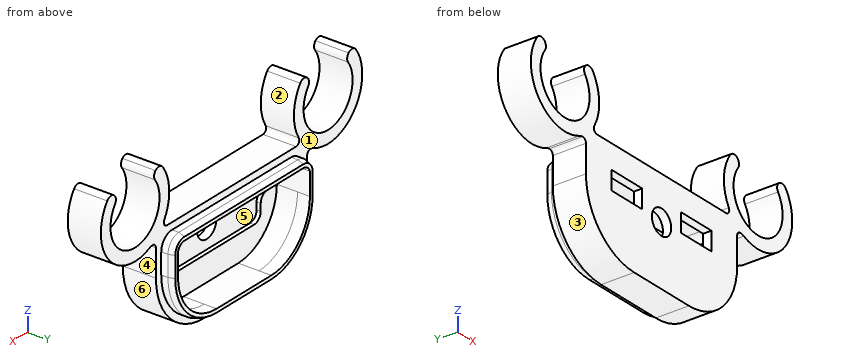
```python
from build123d import *

# Parameters (mm, degrees)
SKETCH1_W               = 47
SKETCH1_H               = 25
BOSS_EXTRUDE1_DEPTH     = 8
SHELL1_T                = -3
SKETCH4_R               = 3
SKETCH4_W               = 9.5
SKETCH4_H               = 4.5
CUT_EXTRUDE4_DEPTH      = 28.793884219
FILLET2_R               = 12
FILLET3_R               = 15
SKETCH5_R               = 7.625
BOSS_EXTRUDE3_DEPTH     = 8
FILLET7_R               = 2
FILLET9_R               = 3
FILLET10_R              = 3
BOSS_EXTRUDE4_DEPTH     = 3
FILLET11_R              = 1
CHAMFER1_SIZE           = 0.5
CHAMFER1_SIZE2          = 1.37373871
CUT_EXTRUDE5_DEPTH      = 10
CUT_EXTRUDE5_DEPTH_BACK = 1
CUT_EXTRUDE6_DEPTH      = 10
FILLET12_R              = 1.5


# Some blends are built 0.0001 mm under size
with BuildPart() as part:
    # Sketch1 → Boss-Extrude1 (new body)
    with BuildSketch(Plane(origin=(0, 0, 0), x_dir=(1, 0, 0), z_dir=(0, 1, 0))):
        Rectangle(SKETCH1_W, SKETCH1_H)
    extrude(amount=BOSS_EXTRUDE1_DEPTH)

    # Shell1
    shell1_openings = [part.faces().sort_by_distance(p)[0] for p in [
        (0, 8, 0),
    ]]
    offset(amount=SHELL1_T, openings=shell1_openings, kind=Kind.INTERSECTION)

    # Sketch4 → Cut-Extrude4 (cut, through all)
    with BuildSketch(Plane.XZ):
        with Locations(Location((0, 2, 0), (0, 0, 270))):
            Circle(SKETCH4_R)
        with Locations((10.75, 4.5)):
            Rectangle(SKETCH4_W, SKETCH4_H)
        with Locations((-10.75, 4.5)):
            Rectangle(SKETCH4_W, SKETCH4_H)
    extrude(amount=-CUT_EXTRUDE4_DEPTH, mode=Mode.SUBTRACT)

    # Fillet2
    fillet2_edges = [part.edges().sort_by_distance(p)[0] for p in [
        (-20.5, 5.5, -9.5),
        (20.5, 5.5, -9.5),
    ]]
    fillet(fillet2_edges, radius=FILLET2_R)

    # Fillet3
    fillet3_edges = [part.edges().sort_by_distance(p)[0] for p in [
        (-23.5, 4, -12.5),
        (23.5, 4, -12.5),
    ]]
    fillet(fillet3_edges, radius=FILLET3_R)

    # Sketch5 → Boss-Extrude3 (add)
    # profile 1 of 2: a face of its own
    with BuildSketch(Plane(origin=(0, 0, 0), x_dir=(1, 0, 0), z_dir=(0, 1, 0))):
        with BuildLine():
            Line((-24.109061312, -10.65763231), (-23.023781022, -9.5))
            Line((-23.023781022, -9.5), (-18.817115042, -9.5))
            Line((-18.817115042, -9.5), (-21.851077989, -12.681958121))
            ThreePointArc((-21.851077989, -12.681958121), (-37.092523941, -27.411177481), (-24.109061312, -10.65763231))
        make_face()
        with Locations(Location((-30, -19.5, 0), (0, 0, 270))):
            Circle(SKETCH5_R, mode=Mode.SUBTRACT)
    # profile 2 of 2: a face of its own
    with BuildSketch(Plane(origin=(0, 0, 0), x_dir=(1, 0, 0), z_dir=(0, 1, 0))):
        with BuildLine():
            Line((21.851077989, -12.681958121), (18.817115042, -9.5))
            Line((18.817115042, -9.5), (23.023781022, -9.5))
            Line((23.023781022, -9.5), (24.109061312, -10.65763231))
            ThreePointArc((24.109061312, -10.65763231), (37.092523941, -27.411177481), (21.851077989, -12.681958121))
        make_face()
        with Locations(Location((30, -19.5, 0), (0, 0, 90))):
            Circle(SKETCH5_R, mode=Mode.SUBTRACT)
    extrude(amount=BOSS_EXTRUDE3_DEPTH)

    # Fillet7
    fillet7_edges = [part.edges().sort_by_distance(p)[0] for p in [
        (-20.5, 5.5, 9.5),
        (20.5, 5.5, 9.5),
    ]]
    fillet(fillet7_edges, radius=FILLET7_R)

    # Fillet9
    # the kernel refuses this fillet: 3 mm, written as the material it adds along each edge
    with BuildSketch(Plane(origin=(-24.109061312, 0, 10.65763231), x_dir=(-0.8731241588548913, 0, -0.48749790073798127), z_dir=(0, 1, 0))) as fillet9_piece_1:
        with BuildLine():
            CenterArc((1.900937986, -2.990768498), FILLET9_R, 94.495982628, 40.36086399)
            Line((-0.215075627, -0.864154666), (-0.2573959, -0.82162239))
            ThreePointArc((-0.2573959, -0.82162239), (-0.165761599, -0.417586273), (-0.058223785, 0.01449106))
            Line((-0.058223785, 0.01449106), (0.004703352, 0.05981537))
            ThreePointArc((0.004703352, 0.05981537), (0.8328852, 0.027305096), (1.661067049, 0.05981537))
            Line((1.661067049, 0.05981537), (1.6657704, 0))
        make_face()
    extrude(amount=8)
    with BuildSketch(Plane(origin=(24.109061312, 0, 10.65763231), x_dir=(-0.6839411288813303, 0, -0.7295372041400846), z_dir=(0, 1, 0))) as fillet9_piece_2:
        with BuildLine():
            CenterArc((2.443120942, -2.566986852), FILLET9_R, 121.167021746, 40.36086399)
            Line((-0.402312981, -1.616457637), (-0.45922166, -1.597447053))
            ThreePointArc((-0.45922166, -1.597447053), (-0.227653258, -0.801634155), (-0.059180564, 0.009882353))
            Line((-0.059180564, 0.009882353), (0, 0.06))
            ThreePointArc((0, 0.06), (0.44525858, 0.06), (0.859465085, 0.051339737))
            Line((0.859465085, 0.051339737), (0.89051716, 0))
        make_face()
    extrude(amount=8)

    # Fillet10
    # the kernel refuses this fillet: 3 mm, written as the material it adds along each edge
    with BuildSketch(Plane(origin=(-21.851077989, 0, 12.681958121), x_dir=(0.6041926909004034, 0, 0.796838247238754), z_dir=(0, 1, 0))) as fillet10_piece_1:
        with BuildLine():
            CenterArc((1.162533412, 2.99655072), FILLET10_R, 246.365543593, 20.886670937)
            Line((-0.040166708, 0.248185312), (-0.064220711, 0.193218004))
            ThreePointArc((-0.064220711, 0.193218004), (-0.07931268, 0.114506887), (-0.059229326, -0.009585769))
            Line((-0.059229326, -0.009585769), (0.002876371, -0.059931014))
            ThreePointArc((0.002876371, -0.059931014), (0.509357423, -0.047783801), (1.015838475, -0.059931014))
            Line((1.015838475, -0.059931014), (1.018714846, 0))
        make_face()
    extrude(amount=8)
    with BuildSketch(Plane(origin=(21.851077989, 0, 12.681958121), x_dir=(-0.6041926909004038, 0, 0.7968382472387535), z_dir=(0, 1, 0))) as fillet10_piece_2:
        with BuildLine():
            CenterArc((1.162533412, -2.99655072), FILLET10_R, 92.74778547, 20.886670937)
            Line((-0.040166708, -0.248185312), (-0.064220711, -0.193218004))
            ThreePointArc((-0.064220711, -0.193218004), (-0.07931268, -0.114506887), (-0.059229326, 0.009585769))
            Line((-0.059229326, 0.009585769), (0.002876371, 0.059931014))
            ThreePointArc((0.002876371, 0.059931014), (0.509357423, 0.047783801), (1.015838475, 0.059931014))
            Line((1.015838475, 0.059931014), (1.018714846, 0))
        make_face()
    extrude(amount=8)

    # Sketch6 → Boss-Extrude4 (add)
    with BuildSketch(Plane(origin=(0, 8, 0), x_dir=(1, 0, 0), z_dir=(0, 1, 0))):
        with BuildLine():
            Line((-21.85, -2.5), (-21.85, -7.5))
            ThreePointArc((-21.85, -7.5), (-20.868807717, -9.868807717), (-18.5, -10.85))
            Line((-18.5, -10.85), (18.5, -10.85))
            ThreePointArc((18.5, -10.85), (20.868807717, -9.868807717), (21.85, -7.5))
            Line((21.85, -7.5), (21.85, -2.5))
            ThreePointArc((21.85, -2.5), (17.939875529, 6.939875529), (8.5, 10.85))
            Line((8.5, 10.85), (-8.5, 10.85))
            ThreePointArc((-8.5, 10.85), (-17.939875529, 6.939875529), (-21.85, -2.5))
        make_face()
        with BuildLine():
            Line((-18.5, -9.5), (18.5, -9.5))
            ThreePointArc((18.5, -9.5), (19.914213562, -8.914213562), (20.5, -7.5))
            Line((20.5, -7.5), (20.5, -2.5))
            ThreePointArc((20.5, -2.5), (16.985281374, 5.985281374), (8.5, 9.5))
            Line((8.5, 9.5), (-8.5, 9.5))
            ThreePointArc((-8.5, 9.5), (-16.985281374, 5.985281374), (-20.5, -2.5))
            Line((-20.5, -2.5), (-20.5, -7.5))
            ThreePointArc((-20.5, -7.5), (-19.914213562, -8.914213562), (-18.5, -9.5))
        make_face(mode=Mode.SUBTRACT)
    extrude(amount=BOSS_EXTRUDE4_DEPTH)

    # Fillet11
    fillet11_edges = [part.edges().sort_by_distance(p)[0] for p in [
        (21.677582872, 4, 12.5),
        (23.5, 4, 10.00796691),
        (-21.677582872, 4, 12.5),
        (-23.5, 4, 10.00796691),
    ]]
    fillet(fillet11_edges, radius=FILLET11_R)

    # Chamfer1
    chamfer1_edges = [part.edges().sort_by_distance(p)[0] for p in [
        (-17.939875529, 11, -6.939875529),
        (-21.85, 11, 5),
        (-20.868807717, 11, 9.868807717),
        (0, 11, 10.85),
        (20.868807717, 11, 9.868807717),
        (21.85, 11, 5),
        (17.939875529, 11, -6.939875529),
        (0, 11, -10.85),
    ]]
    chamfer1_side = [part.faces().sort_by_distance(p)[0] for p in [
        (-21.362088123, 11, 5),
    ]]
    chamfer(chamfer1_edges, length=CHAMFER1_SIZE, length2=CHAMFER1_SIZE2, reference=chamfer1_side[0])

    # Sketch7 → Cut-Extrude5 (cut, two sides: drawn at the far end of the back side and taken through both)
    with BuildSketch(Plane(origin=(0, 3, 0), x_dir=(1, 0, 0), z_dir=(0, 1, 0)).offset(-CUT_EXTRUDE5_DEPTH_BACK)):
        with BuildLine():
            Line((-20.5, -6.75), (-20.5, -2.5))
            Line((-20.5, -2.5), (-17.5, -2.5))
            ThreePointArc((-17.5, -2.5), (-16.085786438, -1.914213562), (-15.5, -0.5))
            Line((-15.5, -0.5), (-15.5, 1.25))
            ThreePointArc((-15.5, 1.25), (-14.914213562, 2.664213562), (-13.5, 3.25))
            Line((-13.5, 3.25), (13.5, 3.25))
            ThreePointArc((13.5, 3.25), (14.914213562, 2.664213562), (15.5, 1.25))
            Line((15.5, 1.25), (15.5, -0.5))
            ThreePointArc((15.5, -0.5), (16.085786438, -1.914213562), (17.5, -2.5))
            Line((17.5, -2.5), (20.5, -2.5))
            Line((20.5, -2.5), (20.5, -6.75))
            Line((20.5, -6.75), (20.5, -8))
            Line((20.5, -8), (-20.5, -8))
            Line((-20.5, -8), (-20.5, -6.75))
        make_face()
    extrude(amount=CUT_EXTRUDE5_DEPTH + CUT_EXTRUDE5_DEPTH_BACK, mode=Mode.SUBTRACT)

    # Sketch8 → Cut-Extrude6 (cut)
    with BuildSketch(Plane.XZ):
        Polygon((-30, 19.5), (-42.679355302, 32.179355302), (-17.320644698, 32.179355302), align=None)
        Polygon((42.679355302, 32.179355302), (17.320644698, 32.179355302), (30, 19.5), align=None)
    extrude(amount=-CUT_EXTRUDE6_DEPTH, mode=Mode.SUBTRACT)

    # Fillet12
    fillet12_edges = [part.edges().sort_by_distance(p)[0] for p in [
        (37.51300955, 4, 27.01300955),
        (35.391689207, 4, 24.891689207),
        (24.608310793, 4, 24.891689207),
        (22.48699045, 4, 27.01300955),
        (-24.608310793, 4, 24.891689207),
        (-22.48699045, 4, 27.01300955),
        (-35.391689207, 4, 24.891689207),
        (-37.51300955, 4, 27.01300955),
    ]]
    fillet(fillet12_edges, radius=FILLET12_R - 0.0001)  # a hair under: the kernel refuses the full size


solid = part.part
```
Here's how the part is built. I have some questions about the finished solid (model axes, mm). Face numbers are marked on the shaded views. A direction names the side the tool comes from. Coordinates: 2 decimals unless noted, no trailing zeros. Loops run counter-clockwise (first coordinate to the right, second up) from the corner with the lowest first, then second, coordinate; pieces in that order, holes last. Notation, with made-up numbers: (-27.75, 49) - (-11.75, 49) arc R14 ccw to (-11.75, 59) - close; hole circle Ø10 at (-9, -27.75). An arc over 180 degrees is marked (long way). Return JSON: item names as keys, results as strings. Group by question number.
Item 1: If we section it at A-A on x = 0: Write out the boundary of the cut face in (y, z), and give its area (3 significant figures).
Item 2: On a 3-axis mill with a long thin cutter (end or side, diameter ignored), from which of +Z, -Z, +X, -X, +Y, -Y can I reach the whole of each face in a straight line? I mean the marked faces 1, 2 and 3. Say none if no direction works.
Item 3: If we section it at C-C on x = 30: Write out the boundary of the cut face in (y, z) (3 decimals), and give its area (3 significant figures).
Item 4: Will these pins go through, and if not, where does the flat tip stop? P1, Ø6, axis at y = 7, z = 5.5, coming from the +X side; P2, Ø1, axis at x = 12.5, y = 1, coming from the +Z side; P3, Ø2, axis at y = 7.5, z = 0, coming from the +X side; P4, Ø13.5, axis at x = -30, z = 19.5, coming from the +Y side.
Item 5: We'd pull the mould along Z, two halves only. Please class the marked faces 4, 5 and 6: +Z half, -Z half, draft (parallel to the pull), parting line (faces both ways), or undercut.
Item 6: If we section it at B-B on z = 21.5: Write out the boundary of the cut face in (x, y), and give its area (3 significant figures).
Item 7: I need wall thicknesses on line 1 (X direction, y = 4.5, z = 19.5) (3 decimals); line 2 (Z direction, x = 9, y = 6.25); line 3 (X direction, y = 4, z = 14.5) (3 decimals). Which ranges of each line are inside material? Lowest first, please. Write a range as from..to.
Calculated:
{
 "1": {"outline": "(0, -12.5) - (8, -12.5) - (8, -10.85) - (9.63, -10.85) - (11, -10.35) - (11, -9.5) - (3, -9.5) - (3, -3.25) - (2, -3.25) - (2, -1) - (0, -1) - close; (0, 5) - (2, 5) - (2, 8) - (3, 8) - (3, 9.5) - (11, 9.5) - (11, 10.35) - (9.63, 10.85) - (8, 10.85) - (8, 12.5) - (0, 12.5) - close", "area": "89.2 mm^2"},
 "2": {"face 1": "+Y", "face 2": "+Y, -Y", "face 3": "-Z, -X, +Y, -Y"},
 "3": {"outline": "(0, 8.875) - (8, 8.875) - (8, 11.875) - (0, 11.875) - close", "area": "24.0 mm^2"},
 "4": {"P1": "stops at x = 23.5", "P2": "stops at z = 12.5", "P3": "stops at x = 23.42", "P4": "passes through"},
 "5": {"face 4": "draft", "face 5": "undercut", "face 6": "-Z half"},
 "6": {"outline": "(-40.44, 0) - (-37.36, 0) - (-37.36, 8) - (-40.44, 8) - close; (-22.64, 0) - (-19.56, 0) - (-19.56, 8) - (-22.64, 8) - close; (19.56, 0) - (22.64, 0) - (22.64, 8) - (19.56, 8) - close; (37.36, 0) - (40.44, 0) - (40.44, 8) - (37.36, 8) - close", "area": "98.5 mm^2"},
 "7": {"line 1": "x = -40.625..-37.625, -22.375..-19.375, 19.375..22.375, 37.625..40.625", "line 2": "z = -12.49..-9.49, 9.5..12.5", "line 3": "x = -39.375..-35.757, -24.243..-20.625, 20.625..24.243, 35.757..39.375"}
}
